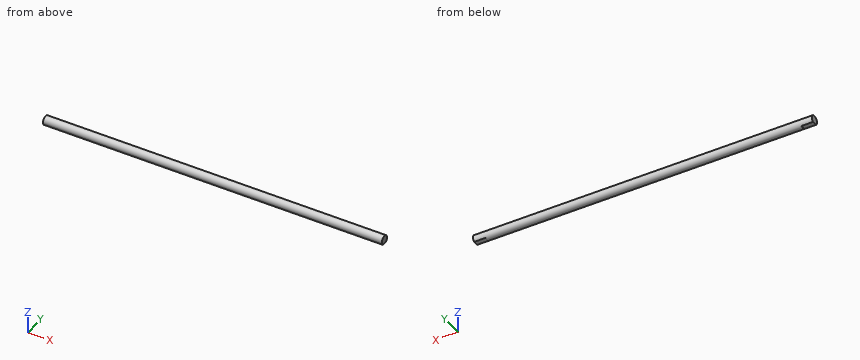
from build123d import *

# Parameters (mm, degrees)
SKETCH_1_R          = 6
EXTRUDE_1_DEPTH     = 460
SKETCH_2_W          = 15.5
SKETCH_2_H          = 1
CUT_EXTRUDE_1_DEPTH = 200


with BuildPart() as part:
    # 草图1 → 凸台-拉伸1 (new body)
    with BuildSketch(Plane(origin=(0, 0, 0), x_dir=(0, 0, -1), z_dir=(1, 0, 0))):
        Circle(SKETCH_1_R)
    extrude(amount=EXTRUDE_1_DEPTH)

    # 草图2 → 切除-拉伸1 (cut, symmetric)
    with BuildSketch(Plane(origin=(0, 0, 0), x_dir=(1, 0, 0), z_dir=(0, 1, 0))):
        with Locations((7.75, 5.5)):
            Rectangle(SKETCH_2_W, SKETCH_2_H)
    cut_extrude_1 = extrude(amount=CUT_EXTRUDE_1_DEPTH, both=True, mode=Mode.SUBTRACT)

    # 镜向1: 切除-拉伸1 across plane
    add(cut_extrude_1.mirror(Plane.ZY.offset(-230)), mode=Mode.SUBTRACT)


solid = part.part
Input: part model. Units: mm. Frame: model coordinates. Round coordinates to 2 decimals unless told otherwise and drop trailing zeros. Order: outer loops, then holes, each group sorted by start corner. A loop starts at its lowest first (then second) coordinate and runs counter-clockwise, first axis right, second up.
1. Pin query (flat end, axial travel): P1, Ø0.8, axis at y = 0.5, z = -5.5, coming from the -X side; P2, Ø5, axis at x = 67, z = -3.5, coming from the +Y side; P3, Ø5.5, axis at x = 8.5, y = -0.5, coming from the -Z side. Return the tip coordinate at first contact, or that it passes through.
The answers:
P1: stops at x = 15.5
P2: stops at y = 5.92
P3: stops at z = -5
2. Material intervals for line 1 (Y direction, x = 265.5, z = -1); line 2 (Y direction, x = 128, z = -0.25); line 3 (Z direction, x = 336.5, y = 0.75), sorted ascending.
The answers:
line 1: y = -5.92 to 5.92
line 2: y = -5.99 to 5.99
line 3: z = -5.95 to 5.95
3. Cut plane B-B, the plane z = -1.5. Output: boundary loops of the cut face in (x, y).
The answers:
outline: (0, -5.81) - (460, -5.81) - (460, 5.81) - (0, 5.81) - close
4. Cut plane A-A, the plane x = 48. Output: boundary loops of the cut face in (y, z), then the cut area to 3 significant figures.
The answers:
outline: circle Ø12 at (0, 0)
area: 113 mm2
